```python
from build123d import *

# Parameters (mm, degrees)
MODEL_R                 = 3.800728286
SALIENTE_EXTRUIR1_DEPTH = 0.1


with BuildPart() as part:
    # Model → Saliente-Extruir1 (new body)
    with BuildSketch(Plane.XY):
        with BuildLine():
            Line((13.692923281, 36.409278797), (9.778554106, 35.797482596))
            Line((9.778554106, 35.797482596), (9.291241734, 35.721318124))
            ThreePointArc((9.291241734, 35.721318124), (6.601579479, 34.038755415), (4.608572881, 31.570309544))
            Line((4.608572881, 31.570309544), (12.45581545, 19.849854112))
            ThreePointArc((12.45581545, 19.849854112), (12.812940227, 17.870349583), (12.922946265, 15.861898697))
            Line((12.922946265, 15.861898697), (13.203519251, 10.044821535))
            Line((13.203519251, 10.044821535), (14.770932303, 7.477024351))
            Line((14.770932303, 7.477024351), (14.770932303, 4.477024351))
            Line((14.770932303, 4.477024351), (14.770932303, 1.777024351))
            Line((14.770932303, 1.777024351), (18.272189759, 1.777024351))
            Line((18.272189759, 1.777024351), (18.272189759, 23.155058368))
            Line((18.272189759, 23.155058368), (33.772189759, 23.155058368))
            Line((33.772189759, 23.155058368), (34.772189759, 23.155058368))
            Line((34.772189759, 23.155058368), (50.272189759, 23.155058368))
            Line((50.272189759, 23.155058368), (50.272189759, 1.777024351))
            Line((50.272189759, 1.777024351), (53.770932303, 1.775742122))
            Line((53.770932303, 1.775742122), (53.770932303, 5.477024351))
            Line((53.770932303, 5.477024351), (54.065641416, 8.331670065))
            Line((54.065641416, 8.331670065), (55.340860267, 10.044821535))
            Line((55.340860267, 10.044821535), (55.55942352, 16.069253716))
            ThreePointArc((55.55942352, 16.069253716), (55.715346099, 17.974760468), (56.088564069, 19.849854112))
            Line((56.088564069, 19.849854112), (63.866724949, 31.491817154))
            ThreePointArc((63.866724949, 31.491817154), (61.853109226, 34.011935883), (59.141967464, 35.759893842))
            Line((59.141967464, 35.759893842), (51.731314314, 36.906395207))
            Line((51.731314314, 36.906395207), (47.893743211, 27.949013218))
            Line((47.893743211, 27.949013218), (34.272189759, 24.431748181))
            Line((34.272189759, 24.431748181), (20.650636308, 27.949013218))
            Line((20.650636308, 27.949013218), (16.81686132, 36.89753459))
            Line((16.81686132, 36.89753459), (13.692923281, 36.409278797))
        make_face()
        with Locations((53.808865901, 26.441300342)):
            Circle(MODEL_R, mode=Mode.SUBTRACT)
    extrude(amount=SALIENTE_EXTRUIR1_DEPTH)


solid = part.part
```
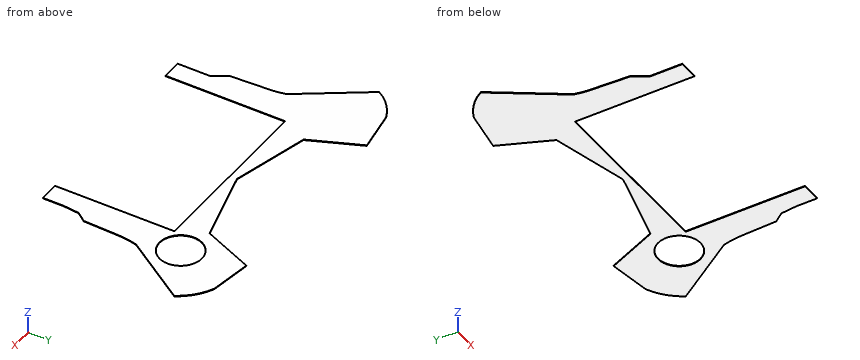
Can you work these out from the model? Positions are in its coordinate system, mm. Coordinates: 2 decimals unless noted, no trailing zeros. Write each loop counter-clockwise with the first axis right and the second up, starting at its lowest first coordinate (ties: lowest second). Pieces come first, ordered by that corner, then holes. Notation, with made-up numbers: M 50,68 L 104,68 A16 cw 104,94 Z; hole C 86,46 d10. An arc over 180 degrees is marked long. Write item = value, one per line. Start each with the question number.
Q1. If we section it at A-A, the plane y = 18: Write out the boundary of the cut face in (x, z), then the cut area to 3 significant figures.
Q2. If we section it at C-C, the plane y = 13: Write out the boundary of the cut face in (x, z).
Q3. If we section it at D-D, the plane x = 43: Write out the boundary of the cut face in (y, z).
Q4. If I drill on L1, parallel to Y at x = 36, z = 0.05; L2, parallel to Y at x = 46, z = 0.05, over which ranges is the centre line in solid material (lowest first)? Write a range as [from, to].
Q5. If we section it at B-B, the plane y = 27: Write out the boundary of the cut face in (x, z), then the cut area to 3 significant figures.
Check sheet entries:
q1.outline = M 12.8,0 L 18.27,0 L 18.27,0.1 L 12.8,0.1 Z; M 50.27,0 L 55.72,0 L 55.72,0.1 L 50.27,0.1 Z
q1.area = 1.09 mm²
q2.outline = M 13.06,0 L 18.27,0 L 18.27,0.1 L 13.06,0.1 Z; M 50.27,0 L 55.45,0 L 55.45,0.1 L 50.27,0.1 Z
q3.outline = M 23.16,0 L 26.69,0 L 26.69,0.1 L 23.16,0.1 Z
q4.L1 = [23.16, 24.88]
q4.L2 = [23.16, 27.46]
q5.outline = M 7.67,0 L 24.33,0 L 24.33,0.1 L 7.67,0.1 Z; M 44.22,0 L 50.05,0 L 50.05,0.1 L 44.22,0.1 Z; M 57.57,0 L 60.87,0 L 60.87,0.1 L 57.57,0.1 Z
q5.area = 2.58 mm²
